Part model, mm, in its own coordinate system. Face numbers are marked on the shaded views. A direction names the side the tool comes from. Round coordinates to 2 decimals unless told otherwise and drop trailing zeros. Loops run counter-clockwise (first coordinate to the right, second up) from the corner with the lowest first, then second, coordinate; pieces in that order, holes last.
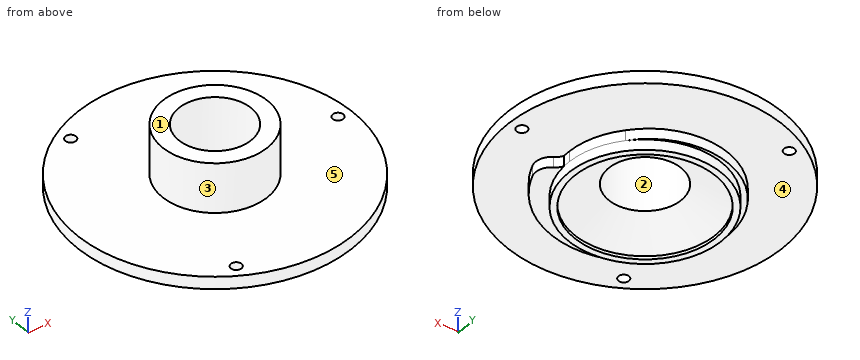
from build123d import *
from build123d.topology import SkipClean

# Parameters (mm, degrees)
SKETCH18_R             = 47.625
CUT_EXTRUDE2_DEPTH     = 5
F_10_CLEARANCE_HOLE1_D = 5.1054
CIRPATTERN1_COUNT      = 3


with BuildPart() as part:
    # Sketch24 → Revolve1 (revolve)
    with BuildSketch(Plane(origin=(0, 0, 0), x_dir=(1, 0, 0), z_dir=(0, 1, 0))):
        Polygon((-37, 81.654237034), (-37, 76.654237034), (-47.625, 76.654237034), (-47.625, 71.654237034), (-66.675, 71.654237034), (-66.675, 65.654237034), (-25.4, 65.654237034), (-25.4, 41.654237034), (-17.5, 41.654237034), (-17.5, 70.627957592), (-34, 80.154237034), (-34, 81.654237034), align=None)
    revolve(axis=Axis((0, 0, -86.654237034), (0, 0, 1)))

    # Sketch18 → Cut-Extrude2 (cut)
    with SkipClean():  # the faces are left unmerged after this step: merging them gives an invalid solid
        with BuildSketch(Plane.XY.offset(-76.654237034)):
            Circle(SKETCH18_R)
            with BuildLine():
                ThreePointArc((36.803517411, -3.8080318), (37.978132396, -5.474504313), (39.552581276, -6.769865934))
                ThreePointArc((39.552581276, -6.769865934), (42.805320101, -10.94498561), (42.554027377, -16.231646763))
                add(Edge.make_bspline(
                    [(28.227591738, 23.920766389), (28.169074611, 23.995894132), (27.726201544, 24.559979405), (26.867938753, 25.590107465), (25.60001603, 26.964989265), (24.261773335, 28.277085961), (22.856314773, 29.522798851), (21.386929147, 30.698682629), (19.85708232, 31.801454876), (18.270409111, 32.828005175), (16.630704717, 33.775403815), (14.941915703, 34.640910073), (13.208130556, 35.421980041), (11.43356985, 36.116273987), (9.622576022, 36.721663214), (7.779602801, 37.236236415), (5.909204301, 37.658305492), (4.016023818, 37.986410831), (2.104782347, 38.219326014), (0.180266852, 38.356061949), (-1.75268168, 38.395870413), (-3.689180377, 38.338246992), (-5.624316777, 38.182933409), (-7.553161251, 37.929919231), (-9.470779522, 37.579442948), (-11.37224525, 37.131992419), (-13.252652651, 36.588304682), (-15.107129112, 35.949365124), (-16.930847778, 35.216406011), (-18.719040078, 34.390904381), (-20.467008144, 33.474579298), (-22.170137115, 32.469388481), (-23.823907266, 31.377524301), (-25.42390596, 30.201409162), (-26.965839357, 28.943690275), (-28.445543888, 27.607233836), (-29.858997424, 26.195118613), (-31.202330147, 24.710628968), (-32.471835063, 23.157247319), (-33.663978152, 21.538646066), (-34.775408104, 19.858679), (-35.802965645, 18.121372202), (-36.743692396, 16.330914471), (-37.594839261, 14.491647299), (-38.353874308, 12.608054401), (-39.018490139, 10.68475085), (-39.586610697, 8.726471825), (-40.056397525, 6.738061006), (-40.426255434, 4.724458642), (-40.694837576, 2.690689328), (-40.861049894, 0.641849508), (-40.924054953, -1.416905249), (-40.883275123, -3.480373184), (-40.738395114, -5.543319447), (-40.489363842, -7.600489337), (-40.13639564, -9.646621653), (-39.679970776, -11.676462103), (-39.120835312, -13.684776759), (-38.460000265, -15.666365517), (-37.698740094, -17.61607551), (-36.838590511, -19.528814477), (-35.881345602, -21.399564006), (-34.829054288, -23.223392663), (-33.684016107, -24.995468936), (-32.44877635, -26.711073982), (-31.126120537, -28.365614138), (-29.719068263, -29.954633155), (-28.230866416, -31.473824138), (-26.664981791, -32.919041144), (-25.025093105, -34.286310417), (-23.315082441, -35.571841228), (-21.53902614, -36.772036288), (-19.701185153, -37.883501708), (-17.805994889, -38.903056478), (-15.85805457, -39.827741435), (-13.862116128, -40.654827709), (-11.823072667, -41.381824596), (-9.745946518, -42.006486871), (-7.635876912, -42.526821485), (-5.498107312, -42.941093656), (-3.337972426, -43.247832311), (-1.160884928, -43.445834888), (1.027678058, -43.534171454), (3.222188708, -43.512188152), (5.417082419, -43.379509955), (7.606771886, -43.136042707), (9.785661288, -42.781974466), (11.948160555, -42.317776118), (14.08869967, -41.74420128), (16.201742982, -41.062285471), (18.281803484, -40.273344558), (20.323457017, -39.378972487), (22.321356376, -38.381038284), (24.27024527, -37.281682345), (26.164972102, -36.083312015), (28.000503535, -34.788596469), (29.77193781, -33.400460899), (31.474517775, -31.92208003), (33.103643596, -30.356870964), (34.654885111, -28.708485383), (36.123993806, -26.980801118), (37.506914359, -25.17791311), (38.799795742, -23.304123775), (39.999001844, -21.363932809), (41.101121576, -19.362026441), (41.938186302, -17.641904891), (42.402189205, -16.588613759), (42.554027377, -16.231646763)],
                    knots=[0.099688645, 0.099688645, 0.099688645, 0.099688645, 0.100798534, 0.108047194, 0.115310927, 0.122589766, 0.12988374, 0.13719288, 0.144517215, 0.151856774, 0.159211583, 0.16658167, 0.173967063, 0.181367786, 0.188783866, 0.196215328, 0.203662198, 0.211124498, 0.218602253, 0.226095488, 0.233604225, 0.241128486, 0.248668296, 0.256223676, 0.263794648, 0.271381234, 0.278983456, 0.286601335, 0.294234891, 0.301884146, 0.309549121, 0.317229835, 0.324926308, 0.332638561, 0.340366614, 0.348110485, 0.355870195, 0.363645762, 0.371437205, 0.379244543, 0.387067795, 0.39490698, 0.402762115, 0.410633219, 0.41852031, 0.426423405, 0.434342523, 0.442277682, 0.450228898, 0.458196189, 0.466179572, 0.474179065, 0.482194684, 0.490226447, 0.498274369, 0.506338468, 0.514418761, 0.522515263, 0.530627991, 0.538756962, 0.546902191, 0.555063694, 0.563241488, 0.571435588, 0.57964601, 0.58787277, 0.596115883, 0.604375364, 0.61265123, 0.620943495, 0.629252175, 0.637577285, 0.64591884, 0.654276855, 0.662651345, 0.671042324, 0.679449808, 0.687873812, 0.696314349, 0.704771435, 0.713245083, 0.721735309, 0.730242127, 0.738765551, 0.747305595, 0.755862273, 0.7644356, 0.77302559, 0.781632256, 0.790255613, 0.798895674, 0.807552454, 0.816225965, 0.824916222, 0.833623239, 0.842347028, 0.851087604, 0.859844979, 0.868619169, 0.877410184, 0.88621804, 0.895042749, 0.903884325, 0.912742781, 0.921618129, 0.930510383, 0.935031581, 0.935031581, 0.935031581, 0.935031581], degree=3))
                ThreePointArc((28.227591738, 23.920766389), (34.737738084, 12.739291693), (37, 0))
                ThreePointArc((37, 0), (36.950846703, -1.906548688), (36.803517411, -3.8080318))
            make_face(mode=Mode.SUBTRACT)
        extrude(amount=CUT_EXTRUDE2_DEPTH, mode=Mode.SUBTRACT)

    # #10 Clearance Hole1 (through all)
    with Locations(Plane(origin=(60.325, 0, -71.654237034), x_dir=(-1, 0, 0), z_dir=(0, 0, -1))):
        with Locations((0, 0)):
            f_10_clearance_hole1 = Hole(F_10_CLEARANCE_HOLE1_D / 2)

    # CirPattern1: #10 Clearance Hole1 ×3 about axis
    with SkipClean():  # the faces are left unmerged after this step: merging them gives an invalid solid
        cirpattern1_axis = Axis((0, 0, 0), (0, 0, 1))
        for i in range(1, CIRPATTERN1_COUNT):
            add(f_10_clearance_hole1.rotate(cirpattern1_axis, i * 360 / CIRPATTERN1_COUNT), mode=Mode.SUBTRACT)


solid = part.part
1) Tool access for the marked faces 4 and 5: list every direction of +Z, -Z, +X, -X, +Y, -Y with a clear straight run to the whole face (end or side of a thin tool).
Values:
face 4: -Z
face 5: +Z
2) Drop flat-ended pins along their axis: pin 1 Ø1.5 at (x, z) = (26.5, -68) entering from +Y; pin 2 Ø6 at (x, y) = (60.325, 0) entering from -Z; pin 3 Ø4 at (y, z) = (-33.5, -64) entering from -X; pin 4 Ø8 at (x, z) = (-49.5, -76) entering from +Y. Give the stop position or say it passes through.
Values:
pin 1: stops at y = 61.5
pin 2: stops at z = -71.65
pin 3: stops at x = -58.29
pin 4: passes through
3) Slice it at D-D, the plane y = 47.5. Give the cut face in (x, z), then the cut area to 3 significant figures.
Values:
outline: (-46.79, -71.65) - (46.79, -71.65) - (46.79, -65.65) - (-46.79, -65.65) - close
area: 561 mm2
4) Slice it at A-A, the plane z = -68.5. Give the number of separate pieces and of enclosed holes in the cut face, then the cut area to 3 significant figures.
Values:
separate pieces: 1
enclosed holes: 4
area: 12,900 mm2
5) Slice it at C-C, the plane x = 54. Give the cut face in (y, z), then the cut area to 3 significant figures.
Values:
outline: (-39.11, -71.65) - (39.11, -71.65) - (39.11, -65.65) - (-39.11, -65.65) - close
area: 469 mm2
6) Wall check: line 1 along Y through (x, z) = (0, -55); line 2 along Y through (x, z) = (0, -80.75). Give the ranges that are in metal, low to high.
Values:
line 1: y = -25.4 to -17.5, 17.5 to 25.4
line 2: y = -37 to -34, 34 to 37
7) Slice it at B-B, the plane z = -45. Give the cut face in (x, y), then the cut area to 3 significant figures.
Values:
outline: circle Ø50.8 at (0, 0); hole circle Ø35 at (0, 0)
area: 1,060 mm2
8) Mould opens along Y. For the marked faces 1, 2 and 3 say: released by +Y, released by -Y, zero draft, split by the parting line, or undercut.
Values:
face 1: zero draft
face 2: undercut
face 3: split by the parting line
